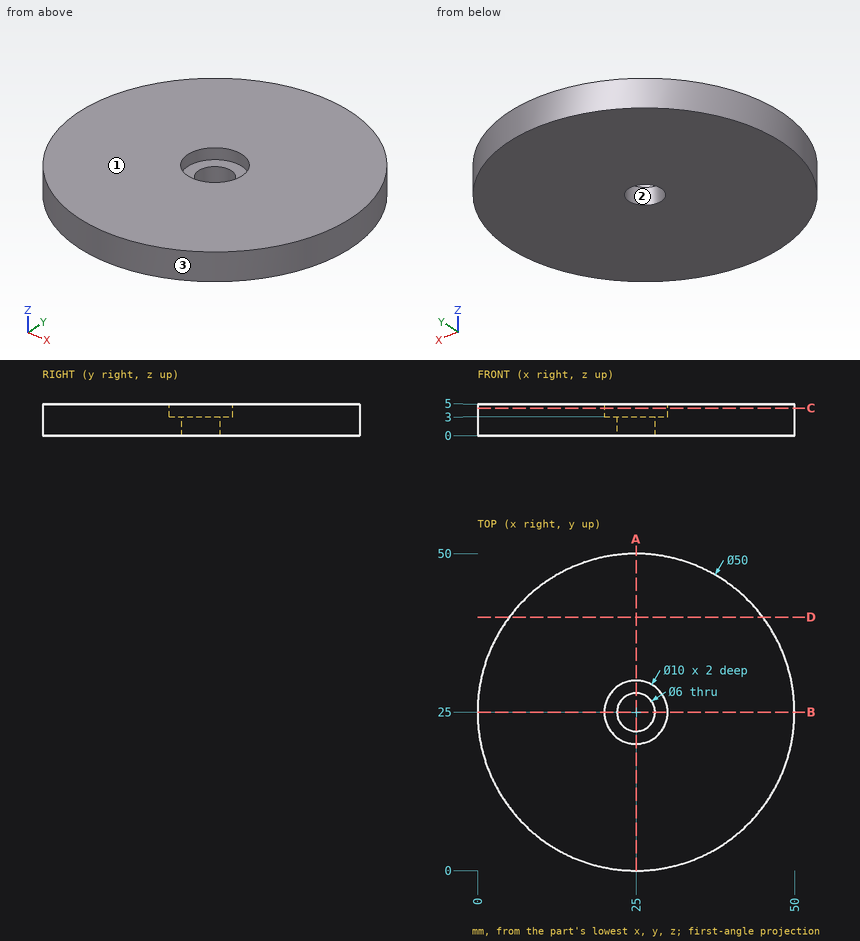
Could you check a few things on this drawing? It's one solid part, dimensions in mm from its lowest x, y, z. Give positions to 0.01 mm unless a question says otherwise; leave off trailing zeros. Write each loop counter-clockwise with the first axis right and the second up, starting at its lowest first coordinate (ties: lowest second). Pieces come first, ordered by that corner, then holes. Notation, with made-up numbers: (-29, 53.25) -> (-9, 53.25) arc R18 cw to (-9, 63.25) -> close; hole circle Ø11 at (-22.75, 24). An arc over 180 degrees is marked (long way). Answer as a JSON object with one key per item and string values.
Q1. Suppose I cut it at C-C on z = 4.35. Write out the boundary of the cut face in (x, y).
Taken from the geometry:
{"outline": "circle Ø50 at (25, 25); hole circle Ø10 at (25, 25)"}
Q2. We'd pull the mould along X, two halves only. Please class the marked faces 1, 2 and 3: released by +X, released by -X, zero draft, split by the parting line, or undercut.
Taken from the geometry:
{"face 1": "zero draft", "face 2": "undercut", "face 3": "split by the parting line"}
Q3. Suppose I cut it at D-D on y = 40. Write out the boundary of the cut face in (x, z), then the cut area to 3 significant figures.
Taken from the geometry:
{"outline": "(5, 0) -> (45, 0) -> (45, 5) -> (5, 5) -> close", "area": "200 mm²"}
Q4. Please list where these lines run through material, in increasing order: L1, parallel to Y at x = 25, z = 1.25; L2, parallel to Y at x = 25, z = 4.2; L3, parallel to X at y = 26, z = 1.55.
Taken from the geometry:
{"L1": "y = 0 to 22, 28 to 50", "L2": "y = 0 to 20, 30 to 50", "L3": "x = 0.02 to 22.17, 27.83 to 49.98"}
Q5. Will these pins go through, and if not, where does the flat tip stop? pin 1 Ø2 at (y, z) = (19, 2.5) entering from -X; pin 2 Ø1.5 at (y, z) = (44, 3.5) entering from -X; pin 3 Ø2 at (y, z) = (9.5, 2.5) entering from -X.
Taken from the geometry:
{"pin 1": "stops at x = 0.51", "pin 2": "stops at x = 7.91", "pin 3": "stops at x = 4.63"}
Q6. Suppose I cut it at A-A on x = 25. Write out the boundary of the cut face in (y, z).
Taken from the geometry:
{"outline": "(0, 0) -> (22, 0) -> (22, 3) -> (20, 3) -> (20, 5) -> (0, 5) -> close; (28, 0) -> (50, 0) -> (50, 5) -> (30, 5) -> (30, 3) -> (28, 3) -> close"}
